Design review of the part shown in the three views and the two pictorial views. Dimensions are in mm from the part's minimum x, y and z. Give positions to 0.01 mm unless a question says otherwise; leave off trailing zeros. Write each loop counter-clockwise with the first axis right and the second up, starting at its lowest first coordinate (ties: lowest second). Pieces come first, ordered by that corner, then holes.
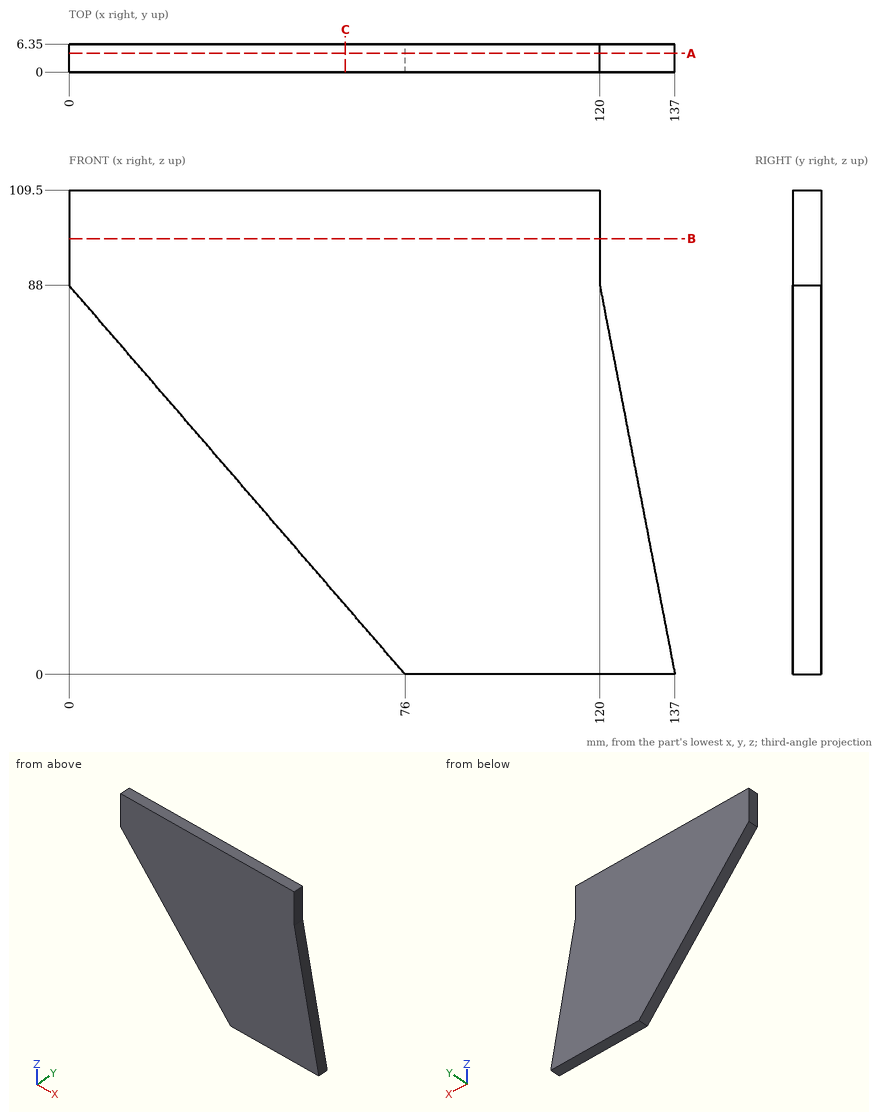
(1) Consider section A-A, the plane y = 4.25. Give the boundary of the cut face in (x, z).
Resolved:
outline: (0, 88) - (76, 0) - (137, 0) - (120, 88) - (120, 109.5) - (0, 109.5) - close
(2) To check wall thickness, follow L1, parallel to X at y = 2, z = 101; L2, parallel to X at y = 2, z = 75; L3, parallel to Z at x = 45, y = 1.75. State the ranges of each line that lie inside material, in increasing order.
Resolved:
L1: x = 0 to 120
L2: x = 11.23 to 122.51
L3: z = 35.89 to 109.5
(3) Consider section C-C, the plane x = 62.5. Give the boundary of the cut face in (y, z), then the cut area to 3 significant figures.
Resolved:
outline: (0, 15.63) - (6.35, 15.63) - (6.35, 109.5) - (0, 109.5) - close
area: 596 mm2
(4) Clearance check with flat-ended pins moving along their axes: P1, Ø1.5, axis at y = 2, z = 89.5, coming from the -X side; P2, Ø1.9, axis at y = 3.5, z = 101, coming from the +X side; P3, Ø1.5, axis at x = 57, y = 4.5, coming from the -Z side. State where each tip first meets the part, or that it passes through.
Resolved:
P1: stops at x = 0
P2: stops at x = 120
P3: stops at z = 21.13
(5) Consider section B-B, the plane z = 98.5. Give the boundary of the cut face in (x, y).
Resolved:
outline: (0, 0) - (120, 0) - (120, 6.35) - (0, 6.35) - close
